Read the model definition and answer for the solid it produces. Units are mm, in the model's axes. A direction names the side the tool comes from. Give positions to 0.01 mm unless a question says otherwise; leave off trailing zeros. Loops run counter-clockwise (first coordinate to the right, second up) from the corner with the lowest first, then second, coordinate; pieces in that order, holes last. Notation, with made-up numbers: (30, 73.25) -> (89, 73.25) arc R10 cw to (89, 88.25) -> close; hole circle Ø4 at (46.5, 8.5). An arc over 180 degrees is marked (long way). Return JSON: item names as keys, results as strings. Group by question number.
Autodesk Inventor part; units mm, degrees
ref_plane "YZ Plane" through (0, 0, 0) normal (1, 0, 0) x (0, 1, 0)
ref_plane "XZ Plane" through (0, 0, 0) normal (0, 1, 0) x (-1, 0, 0)
ref_plane "XY Plane" through (0, 0, 0) normal (0, 0, 1) x (1, 0, 0)
ref_plane "Work Plane1" through (0, 0, 0) normal (0, 0, 1) x (1, 0, 0)
sketch "Sketch1" plane through (0, 0, 0) normal (0, 0, 1) x (1, 0, 0)
  arc A0 (-74.415, -11.0527) -> (-74.415, -5.9883) centre (-76.6839, -8.5205) ccw
  line L0 (-74.415, -11.3137) -> (-74.415, -11.0527)
  line L1 (30, -11.3137) -> (-74.415, -11.3137)
  line L2 (30, 11.3137) -> (30, -11.3137)
  line L3 (25, 11.3137) -> (30, 11.3137)
  line L4 (0, 11.3137) -> (25, 11.3137)
  line L5 (-25, 11.3137) -> (0, 11.3137)
  line L6 (-30, 11.3137) -> (-25, 11.3137)
  line L7 (-30, 16.3137) -> (-30, 11.3137)
  line L8 (-30, 24.6863) -> (-30, 16.3137)
  line L9 (-74.415, 24.6863) -> (-30, 24.6863)
  line L10 (-74.415, -5.9883) -> (-74.415, 24.6863)
  line L11 (-72.2851, 17.6802) -> (-37.2851, 17.6802)
  line L12 (-37.2851, 17.6802) -> (-37.2851, -7.3198)
  line L13 (-37.2851, -7.3198) -> (-72.2851, -7.3198)
  line L14 (-72.2851, -7.3198) -> (-72.2851, 17.6802)
  point P0 (0, 0)
  dimension "d0" = 35
  dimension "d1" = 25
extrude "Extrusion1" add sketch "Sketch1" along normal blind 2 contours L11 L12 L13 L14
sketch "Sketch2" plane through (0, 0, 2) normal (0, 0, 1) x (1, 0, 0)
  line L0 (-37.2851, 17.6802) -> (-72.2851, 17.6802)
  line L1 (-72.2851, 17.6802) -> (-72.2851, -7.3198)
  line L2 (-72.2851, -7.3198) -> (-37.2851, -7.3198)
  line L3 (-37.2851, -7.3198) -> (-37.2851, 17.6802)
  line L4 (-38.2851, 16.6802) -> (-71.2851, 16.6802)
  line L5 (-71.2851, 16.6802) -> (-71.2851, -6.3198)
  line L6 (-71.2851, -6.3198) -> (-38.2851, -6.3198)
  line L7 (-38.2851, -6.3198) -> (-38.2851, 16.6802)
  point P0 (0, 0)
  dimension "d4" = 1
extrude "Extrusion2" add sketch "Sketch2" along normal blind 18
sketch "Sketch3" plane through (-72.2851, -7.3198, 0) normal (-1, 0, 0) x (0, 0, 1)
  line L0 (0, 0) -> (0, 25)
  line L1 (0, 0) -> (20, 0)
  line L2 (20, 25) -> (20, 0)
  line L3 (0, 25) -> (20, 25)
  line L4 (3.37, 23.0819) -> (15.37, 23.0819)
  line L5 (15.37, 23.0819) -> (15.37, 11.0819)
  line L6 (15.37, 11.0819) -> (3.37, 11.0819)
  line L7 (3.37, 11.0819) -> (3.37, 23.0819)
  line L8 (3.37, 23.0819) -> (15.37, 11.0819) construction
  line L9 (15.37, 23.0819) -> (3.37, 11.0819) construction
  point P0 (0, 7.3198)
  point P1 (9.37, 17.0819)
  dimension "d7" = 12
  dimension "d8" = 12
extrude "Extrusion3" cut sketch "Sketch3" against normal blind 15 contours L4 L5 L6 L7
sketch "Sketch4" plane through (-72.2851, 17.6802, 0) normal (0, 1, 0) x (1, 0, 0)
  line L0 (0, 0) -> (35, 0)
  line L1 (0, 0) -> (0, -20)
  line L2 (35, -20) -> (0, -20)
  line L3 (35, 0) -> (35, -20)
  line L4 (17.1417, -3.37) -> (5.1417, -3.37)
  line L5 (5.1417, -3.37) -> (5.1417, -15.37)
  line L6 (5.1417, -15.37) -> (17.1417, -15.37)
  line L7 (17.1417, -15.37) -> (17.1417, -3.37)
  line L8 (17.1417, -3.37) -> (5.1417, -15.37) construction
  line L9 (5.1417, -3.37) -> (17.1417, -15.37) construction
  point P0 (72.2851, 0)
  point P1 (11.1417, -9.37)
  point P2 (0, -3.37)
  dimension "d11" = 12
  dimension "d12" = 12
  dimension "d15" = 0
extrude "Extrusion4" cut sketch "Sketch4" against normal through all contours L7 L6 L5 L4
fillet "Fillet1" radius 2 7 edges at (-71.2851, 5.1802, 2) (-54.7851, 16.6802, 2) (-38.2851, 5.1802, 2) (-54.7851, -6.3198, 2) (-38.2851, -6.3198, 11) (-71.2851, -6.3198, 11) (-38.2851, 16.6802, 11)
properties part number "10_MiniSPIM_Samplechamber"
1. Section B-B on y = 4.25 is taken. Determine the outline of the cut face in (x, z), then the cut area to 3 significant figures.
2. Section D-D on y = 0.75 is taken. Determine the outline of the cut face in (x, z).
3. Section C-C on x = -57.5 is taken. Determine the outline of the cut face in (y, z), then the cut area to 3 significant figures.
4. Which of the six approach directions +Z, -Z, +X, -X, +Y, -Y give full straight-line access (tool end or side, diameter ignored) to faces 4 (the flat face through (-54.5, -7.32, 9.9)), 5 (the flat face through (-61, -7, 3.37)), 6 (the cylindrical face through (-70.684, -5.749, 11.888)), 7 (the flat face through (-72, 10, 3.37))?
5. Determine the mould class of faces 1 (the flat face through (-72, 3.762, 9)), 2 (the flat face through (-56, -7, 20)), 3 (the flat face through (-51, 17.68, 10)) for opening direction Z: pulls with the +Z half, pulls with the -Z half, needs draft (parallel to the pull), parting line crosses it, or undercut.
6. Straight lines are drawn through the part: line 1 (Y direction, x = -43, z = 16.75); line 2 (X direction, y = -2.75, z = 4.25); line 3 (Z direction, x = -69, y = 3.5). For each, find the intervals that lie inside material, in ascending order. Write a range as from..to.
7. Section A-A on z = 14.5 is taken. Determine the outline of the cut face in (x, y), then the cut area to 3 significant figures.
8. A flat-ended cylindrical pin translates along its axis: pin 1 Ø4 at (x, y) = (-50.5, 2.5) entering from +Z. Find the tip coordinate at first contact, or state that the pin passes through.
Completed:
{
 "1": {"outline": "(-72.29, 0) -> (-37.29, 0) -> (-37.29, 20) -> (-38.29, 20) -> (-38.29, 4) arc R2 cw to (-40.29, 2) -> (-69.29, 2) arc R2 cw to (-71.18, 3.37) -> (-72.29, 3.37) -> close; (-72.29, 15.37) -> (-71.29, 15.37) -> (-71.29, 20) -> (-72.29, 20) -> close", "area": "95.7 mm²"},
 "2": {"outline": "(-72.29, 0) -> (-37.29, 0) -> (-37.29, 20) -> (-38.29, 20) -> (-38.29, 4) arc R2 cw to (-40.29, 2) -> (-69.29, 2) arc R2 cw to (-71.29, 4) -> (-71.29, 20) -> (-72.29, 20) -> close"},
 "3": {"outline": "(-7.32, 0) -> (17.68, 0) -> (17.68, 3.37) -> (16.58, 3.37) arc R2 cw to (14.68, 2) -> (-4.32, 2) arc R2 cw to (-6.22, 3.37) -> (-7.32, 3.37) -> close; (-7.32, 15.37) -> (-6.32, 15.37) -> (-6.32, 20) -> (-7.32, 20) -> close; (16.68, 15.37) -> (17.68, 15.37) -> (17.68, 20) -> (16.68, 20) -> close", "area": "63.7 mm²"},
 "4": {"face 4": "+Z, -Z, +X, -X, -Y", "face 5": "+Y, -Y", "face 6": "+Z", "face 7": "-X"},
 "5": {"face 1": "undercut", "face 2": "pulls with the +Z half", "face 3": "needs draft"},
 "6": {"line 1": "y = -7.32..-6.32, 16.68..17.68", "line 2": "x = -72.29..-71.29, -38.29..-37.29", "line 3": "z = 0..2"},
 "7": {"outline": "(-72.29, -7.32) -> (-67.14, -7.32) -> (-67.14, -6.32) -> (-69.29, -6.32) arc R2 cw to (-71.29, -4.32) -> (-71.29, 3.76) -> (-72.29, 3.76) -> close; (-72.29, 15.76) -> (-71.29, 15.76) -> (-71.29, 16.68) -> (-67.14, 16.68) -> (-67.14, 17.68) -> (-72.29, 17.68) -> close; (-55.14, -7.32) -> (-37.29, -7.32) -> (-37.29, 17.68) -> (-55.14, 17.68) -> (-55.14, 16.68) -> (-40.29, 16.68) arc R2 cw to (-38.29, 14.68) -> (-38.29, -4.32) arc R2 cw to (-40.29, -6.32) -> (-55.14, -6.32) -> close", "area": "82.6 mm²"},
 "8": {"pin 1": "stops at z = 2"}
}
